Geometry: final body of the model. Coordinates: model frame, mm. Face numbers are marked on the shaded views. A direction names the side the tool comes from. Round coordinates to 2 decimals unless told otherwise and drop trailing zeros. Order: outer loops, then holes, each group sorted by start corner. A loop starts at its lowest first (then second) coordinate and runs counter-clockwise, first axis right, second up. Notation, with made-up numbers: (51.25, -31) -> (104.25, -31) arc R18 cw to (104.25, -23) -> close; hole circle Ø5 at (61, 85). An arc over 180 degrees is marked (long way). Put each result on its own line as item: value.
```python
from build123d import *

# Parameters (mm, degrees)
F0_R     = 12.25
F1_DEPTH = 30
F2_R     = 12.25
F2_R_2   = 9.525
F3_DEPTH = 10
F4_DEPTH = 10
F5_R     = 9.99999


# Not quite as in the source:
# - a fillet or chamfer is up to 0.001 mm smaller than in the source, because OpenCascade refuses the exact size


with BuildPart() as f1:
    # F0 (on Top) → F1 (new body)
    with BuildSketch(Plane.XY):
        Circle(F0_R)
    extrude(amount=F1_DEPTH)

    # F2 (on face) → F3 (cut)
    with BuildSketch(Plane(origin=(0, 0, 0), x_dir=(1, 0, 0), z_dir=(0, 0, -1))):
        Circle(F2_R)
        Circle(F2_R_2, mode=Mode.SUBTRACT)
    extrude(amount=-F3_DEPTH, mode=Mode.SUBTRACT)

    # F4 (cut): a face of the model
    f4_faces = [f1.faces().sort_by_distance(p)[0] for p in [
        (-11.9035176772, 0, 10),
    ]]
    extrude(f4_faces, amount=-F4_DEPTH, mode=Mode.SUBTRACT)

    # F5 (radius 10 in the source; OpenCascade refuses exactly that, so slightly less here)
    f5_edges = [f1.edges().sort_by_distance(p)[0] for p in [
        (-12.25, 0, 30),
    ]]
    fillet(f5_edges, radius=F5_R)


solid = f1.part
```
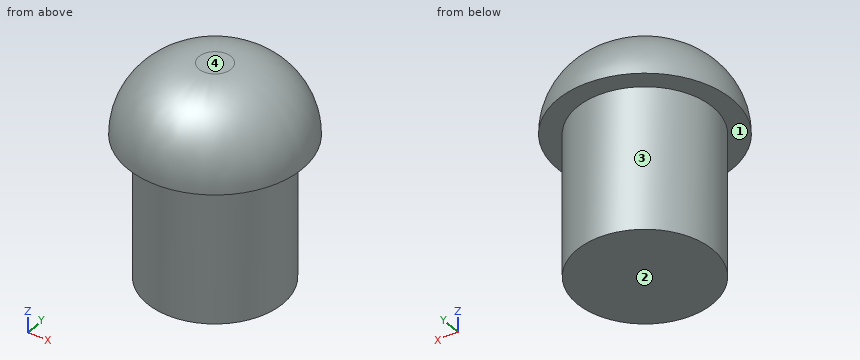
1. Set-up query: the marked faces 1 and 2. Return all of +Z, -Z, +X, -X, +Y, -Y with unobstructed straight access to the full face (end or side cutting, diameter ignored); none if empty.
Ans:
face 1: -Z
face 2: -Z, +X, -X, +Y, -Y
2. Cut plane A-A on z = 4. Return loops of the section in (x, y) (3 decimals).
Ans:
outline: circle Ø19.05 at (0, 0)
3. Contact query for flat-ended pins moving along their axis: P1, Ø12, axis at y = 5.5, z = 7.5, coming from the -X side (3 decimals); P2, Ø8, axis at x = -7, z = 24.5, coming from the -Y side; P3, Ø5, axis at x = 8.5, z = 19.5, coming from the -Y side. Output: stop coordinate, or through.
Ans:
P1: x = -9.525
P2: y = -11.41
P3: y = -10.65
4. Draft query along X for the marked faces 3 and 4. Return one class per face: +X half, -X half, draft (parallel to the pull), parting line (faces both ways), or undercut.
Ans:
face 3: parting line
face 4: draft
5. Material intervals for probe 1 along Z at (x, y) = (2, -1.75); probe 2 along Y at (x, z) = (-0.25, 10.75); probe 3 along Y at (x, z) = (5.75, 12), sorted ascending.
Ans:
probe 1: 0 to 29.99
probe 2: -9.52 to 9.52
probe 3: -7.59 to 7.59
